Could you check a few things on this model? Use its own coordinates, in mm. Coordinates: 2 decimals unless noted, no trailing zeros. Order: outer loops, then holes, each group sorted by start corner. A loop starts at its lowest first (then second) coordinate and runs counter-clockwise, first axis right, second up. Notation, with made-up numbers: (13.5, 65) - (72.5, 65) arc R36 cw to (72.5, 101) - close; hole circle Ø11 at (-34.5, 40). An arc over 180 degrees is marked (long way). One line per item, written item: value.
from build123d import *

# Parameters (mm, degrees)
SKETCH89_R          = 20
SKETCH89_R_2        = 0.836
BOSS_EXTRUDE1_DEPTH = 1.5
BOSS_EXTRUDE2_DEPTH = 2


with BuildPart() as part:
    # Sketch89 → Boss-Extrude1 (new body)
    with BuildSketch(Plane(origin=(0, 32.096297607, 0), x_dir=(1, 0, 0), z_dir=(0, 1, 0))):
        with BuildLine():
            Line((-6.77197393, 31.12758978), (-2.40961654, 31.701905026))
            ThreePointArc((-2.40961654, 31.701905026), (36.88994717, 1.546289176), (6.73433132, -37.753274534))
            Line((6.73433132, -37.753274534), (2.37197393, -38.32758978))
            ThreePointArc((2.37197393, -38.32758978), (-36.92758978, -8.17197393), (-6.77197393, 31.12758978))
        make_face()
        with Locations(Location((-0.018821305, -3.312842377, 0), (0, 0, 270))):
            Circle(SKETCH89_R, mode=Mode.SUBTRACT)
        with Locations(Location((3.247890703, -28.125983544, 0), (0, 0, 270))):
            Circle(SKETCH89_R_2, mode=Mode.SUBTRACT)
        with Locations(Location((-3.285533313, 21.500298789, 0), (0, 0, 270))):
            Circle(SKETCH89_R_2, mode=Mode.SUBTRACT)
    extrude(amount=BOSS_EXTRUDE1_DEPTH)

    # Sketch90 → Boss-Extrude2 (add)
    with BuildSketch(Plane.XZ.offset(-32.096297607)):
        Polygon((1.066712008, 28.413141166), (0.414081046, 23.45591686), (-1.073086246, 23.651706148), (-0.420455285, 28.608930455), align=None)
        Polygon((5.429069398, 27.838825921), (4.776438436, 22.881601614), (6.263605729, 22.685812325), (6.91623669, 27.643036632), align=None)
        Polygon((-0.451723656, -16.830232105), (-1.104354617, -21.787456412), (0.382812675, -21.9832457), (1.035443636, -17.026021394), align=None)
        Polygon((-5.466712008, -21.213141166), (-4.814081046, -16.25591686), (-6.301248339, -16.060127571), (-6.9538793, -21.017351878), align=None)
    extrude(amount=BOSS_EXTRUDE2_DEPTH)


solid = part.part
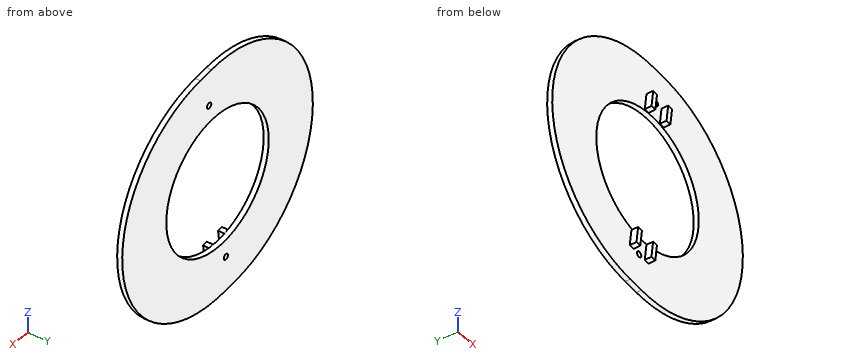
Item 1: I want a section at A-A on y = 31.45. Please give me the cut outline in (x, z), then the cut area to 3 significant figures.
Conclusion:
outline: (-6.95, -21.02) - (-5.47, -21.21) - (-4.81, -16.26) - (-6.3, -16.06) - close; (-1.1, -21.79) - (0.38, -21.98) - (1.04, -17.03) - (-0.45, -16.83) - close; (-1.07, 23.65) - (0.41, 23.46) - (1.07, 28.41) - (-0.42, 28.61) - close; (4.78, 22.88) - (6.26, 22.69) - (6.92, 27.64) - (5.43, 27.84) - close
area: 30.0 mm²
Item 2: I want a section at B-B on z = 21. Please give me the cut outline in (x, y), then the cut area to 3 significant figures.
Conclusion:
outline: (-32.6, 32.1) - (-9.36, 32.1) - (-9.36, 33.6) - (-32.6, 33.6) - close; (9.32, 32.1) - (32.23, 32.1) - (32.23, 33.6) - (9.32, 33.6) - close
area: 69.2 mm²
Item 3: I'm going to push flat-ended pins straight in: pin 1 Ø2.5 at (x, z) = (3.25, 28.13) entering from +Y; pin 2 Ø2.5 at (x, z) = (-3.29, -21.5) entering from -Y; pin 3 Ø1 at (y, z) = (32.5, -20) entering from +X; pin 4 Ø2 at (x, y) = (4.5, 32.5) entering from -Z. Where does each tip first touch, or does it pass through?
Conclusion:
pin 1: y = 33.6
pin 2: y = 32.1
pin 3: x = 28.99
pin 4: z = -31.98
Item 4: I want a section at D-D on x = -30. Please give me the cut outline in (y, z).
Conclusion:
outline: (32.1, -17.71) - (33.6, -17.71) - (33.6, 24.91) - (32.1, 24.91) - close
Item 5: If I drill on probe 1 along Y at (x, z) = (-13, 32); probe 2 along Z at (x, y) = (15, 32.95); probe 3 along X at (y, z) = (32.7, 12), over which ranges is the centre line in solid material (lowest first)?
Conclusion:
probe 1: 32.1 to 33.6
probe 2: -29.56 to -9.89, 16.52 to 35.62
probe 3: -36.21 to -18.03, 18 to 36.02
Item 6: I want a section at C-C on x = -10.5. Please give me the cut outline in (y, z), then the cut area to 3 significant figures.
Conclusion:
outline: (32.1, -30.43) - (33.6, -30.43) - (33.6, -13.72) - (32.1, -13.72) - close; (32.1, 20.35) - (33.6, 20.35) - (33.6, 37.63) - (32.1, 37.63) - close
area: 51.0 mm²
